Design review of the part built by this model. Coordinates are the model's own, in mm. A direction names the side the tool comes from. Give positions to 0.01 mm unless a question says otherwise; leave off trailing zeros. Write each loop counter-clockwise with the first axis right and the second up, starting at its lowest first coordinate (ties: lowest second). Pieces come first, ordered by that corner, then holes.
```python
from build123d import *

# Parameters (mm, degrees)
BOSS_EXTRUDE1_DEPTH = 14.478
BOSS_EXTRUDE2_DEPTH = 66.04
SKETCH3_W           = 80.518
SKETCH3_H           = 1.477027813
BOSS_EXTRUDE3_DEPTH = 1.524
SKETCH4_W           = 80.518
SKETCH4_H           = 1.559652671
CUT_EXTRUDE1_DEPTH  = 1.524
CUT_EXTRUDE3_DEPTH  = 14.478
CUT_EXTRUDE6_DEPTH  = 20.066


with BuildPart() as part:
    # Sketch1 → Boss-Extrude1 (new body)
    with BuildSketch(Plane.XY):
        with BuildLine():
            Line((-72.819716666, 29.55445925), (-5.08, 29.55445925))
            ThreePointArc((-5.08, 29.55445925), (-1.487897552, 28.066561699), (0, 24.47445925))
            Line((0, 24.47445925), (0, -4.589051483))
            ThreePointArc((0, -4.589051483), (-1.487897552, -8.181153932), (-5.08, -9.669051483))
            Line((-5.08, -9.669051483), (-72.819716666, -9.669051483))
            ThreePointArc((-72.819716666, -9.669051483), (-76.411819114, -8.181153932), (-77.899716666, -4.589051483))
            Line((-77.899716666, -4.589051483), (-77.899716666, 24.47445925))
            ThreePointArc((-77.899716666, 24.47445925), (-76.411819114, 28.066561699), (-72.819716666, 29.55445925))
        make_face()
        with BuildLine():
            Line((-65.339884386, 23.351671506), (-12.012527478, 23.351671506))
            ThreePointArc((-12.012527478, 23.351671506), (-8.42042503, 21.863773955), (-6.932527478, 18.271671506))
            Line((-6.932527478, 18.271671506), (-6.932527478, 3.07321573))
            ThreePointArc((-6.932527478, 3.07321573), (-8.42042503, -0.518886719), (-12.012527478, -2.00678427))
            Line((-12.012527478, -2.00678427), (-65.339884386, -2.00678427))
            ThreePointArc((-65.339884386, -2.00678427), (-68.931986835, -0.518886719), (-70.419884386, 3.07321573))
            Line((-70.419884386, 3.07321573), (-70.419884386, 18.271671506))
            ThreePointArc((-70.419884386, 18.271671506), (-68.931986835, 21.863773955), (-65.339884386, 23.351671506))
        make_face(mode=Mode.SUBTRACT)
    extrude(amount=BOSS_EXTRUDE1_DEPTH)

    # Sketch2 → Boss-Extrude2 (add)
    with BuildSketch(Plane(origin=(0, 0, 0), x_dir=(-1, 0, 0), z_dir=(0, 0, -1))):
        with BuildLine():
            Line((5.08, 29.55445925), (72.819716666, 29.55445925))
            ThreePointArc((72.819716666, 29.55445925), (76.411819114, 28.066561699), (77.899716666, 24.47445925))
            Line((77.899716666, 24.47445925), (77.899716666, -4.589051483))
            ThreePointArc((77.899716666, -4.589051483), (76.411819114, -8.181153932), (72.819716666, -9.669051483))
            Line((72.819716666, -9.669051483), (5.08, -9.669051483))
            ThreePointArc((5.08, -9.669051483), (1.487897552, -8.181153932), (0, -4.589051483))
            Line((0, -4.589051483), (0, 24.47445925))
            ThreePointArc((0, 24.47445925), (1.487897552, 28.066561699), (5.08, 29.55445925))
        make_face()
    extrude(amount=BOSS_EXTRUDE2_DEPTH)

    # Sketch3 → Boss-Extrude3 (add)
    with BuildSketch(Plane.ZY.offset(77.899716666)):
        with Locations((-25.781, 23.735945344)):
            Rectangle(SKETCH3_W, SKETCH3_H)
    extrude(amount=-BOSS_EXTRUDE3_DEPTH)

    # Sketch4 → Cut-Extrude1 (cut)
    with BuildSketch(Plane.ZY.offset(77.899716666)):
        with Locations((-25.781, 23.694632915)):
            Rectangle(SKETCH4_W, SKETCH4_H)
    extrude(amount=-CUT_EXTRUDE1_DEPTH, mode=Mode.SUBTRACT)

    # Sketch8 → Cut-Extrude3 (cut)
    with BuildSketch(Plane(origin=(0, 0.399775278, -66.04), x_dir=(-1, 0, 0), z_dir=(0, 0, -1))):
        with BuildLine():
            Line((13.813270209, 22.173227648), (64.646012904, 22.173227648))
            ThreePointArc((64.646012904, 22.173227648), (68.238115352, 20.685330097), (69.726012904, 17.093227648))
            Line((69.726012904, 17.093227648), (69.726012904, 3.751436885))
            ThreePointArc((69.726012904, 3.751436885), (68.238115352, 0.159334436), (64.646012904, -1.328563115))
            Line((64.646012904, -1.328563115), (13.813270209, -1.328563115))
            ThreePointArc((13.813270209, -1.328563115), (10.22116776, 0.159334436), (8.733270209, 3.751436885))
            Line((8.733270209, 3.751436885), (8.733270209, 17.093227648))
            ThreePointArc((8.733270209, 17.093227648), (10.22116776, 20.685330097), (13.813270209, 22.173227648))
        make_face()
    extrude(amount=-CUT_EXTRUDE3_DEPTH, mode=Mode.SUBTRACT)

    # Sketch10 → Cut-Extrude6 (cut)
    with BuildSketch(Plane(origin=(0, 29.55445925, 6.792687041), x_dir=(1, 0, 0), z_dir=(0, 1, 0))):
        with BuildLine():
            Line((-65.795513853, 57.457874707), (-12.761974665, 57.457874707))
            ThreePointArc((-12.761974665, 57.457874707), (-9.169872217, 55.969977155), (-7.681974665, 52.377874707))
            Line((-7.681974665, 52.377874707), (-7.681974665, 11.913822303))
            ThreePointArc((-7.681974665, 11.913822303), (-9.169872217, 8.321719854), (-12.761974665, 6.833822303))
            Line((-12.761974665, 6.833822303), (-65.795513853, 6.833822303))
            ThreePointArc((-65.795513853, 6.833822303), (-69.387616301, 8.321719854), (-70.875513853, 11.913822303))
            Line((-70.875513853, 11.913822303), (-70.875513853, 52.377874707))
            ThreePointArc((-70.875513853, 52.377874707), (-69.387616301, 55.969977155), (-65.795513853, 57.457874707))
        make_face()
    extrude(amount=-CUT_EXTRUDE6_DEPTH, mode=Mode.SUBTRACT)


solid = part.part
```
(1) To check wall thickness, follow L1, parallel to Z at x = -61, y = 26; L2, parallel to X at y = 11, z = -18.5; L3, parallel to Y at x = -38.5, z = 5. State the ranges of each line that lie inside material, in increasing order.
Resolved:
L1: z = -66.04 to -50.67, -0.04 to 14.48
L2: x = -77.9 to -70.88, -7.68 to 0
L3: y = -9.67 to -2.01, 23.35 to 29.55
(2) Tool access review of faces 1 (the face through (-68.198, 21.124, -58.902)), 2 (the face through (-8.4, -0.5, 7.1)), 3 (the face through (-69.35, 19.66, -1.49)): name each direction out of +Z, -Z, +X, -X, +Y, -Y from which nothing blocks a thin tool from reaching the whole face with its end or side.
Resolved:
face 1: -Z
face 2: +Z
face 3: +Y
(3) Consider section C-C, the plane x = -55. Give the boundary of the cut face in (y, z).
Resolved:
outline: (-9.67, -66.04) - (-0.93, -66.04) - (-0.93, -51.56) - (22.57, -51.56) - (22.57, -66.04) - (29.55, -66.04) - (29.55, -50.67) - (9.49, -50.67) - (9.49, -0.04) - (29.55, -0.04) - (29.55, 14.48) - (23.35, 14.48) - (23.35, 0) - (-2.01, 0) - (-2.01, 14.48) - (-9.67, 14.48) - close
(4) Consider section A-A, the plane z = -19. Give the boundary of the cut face in (x, y).
Resolved:
outline: (-77.9, -4.59) arc R5.08 ccw to (-72.82, -9.67) - (-5.08, -9.67) arc R5.08 ccw to (0, -4.59) - (0, 24.47) arc R5.08 ccw to (-5.08, 29.55) - (-7.68, 29.55) - (-7.68, 9.49) - (-70.88, 9.49) - (-70.88, 29.55) - (-72.82, 29.55) arc R5.08 ccw to (-77.9, 24.47) - (-76.38, 24.47) - (-76.38, 22.91) - (-77.9, 22.91) - close
(5) Consider section D-D, the plane y = 0.5. Give the boundary of the cut face in (x, z), then the cut area to 3 significant figures.
Resolved:
outline: (-77.9, -66.04) - (-68.18, -66.04) - (-68.18, -51.56) - (-10.28, -51.56) - (-10.28, -66.04) - (0, -66.04) - (0, 14.48) - (-7.63, 14.48) - (-7.63, 0) - (-69.72, 0) - (-69.72, 14.48) - (-77.9, 14.48) - close
area: 4,540 mm2
(6) Clearance check with flat-ended pins moving along their axes: P1, Ø4, axis at x = -64, y = 9.5, coming from the -Z side; P2, Ø4, axis at x = -45, z = -35, coming from the +Y side; P3, Ø1.2, axis at x = -77, z = -20, coming from the -Y side. State where each tip first meets the part, or that it passes through.
Resolved:
P1: stops at z = -51.56
P2: stops at y = 9.49
P3: stops at y = -8.19
(7) Mouldability with a two-part tool opening along Y and no side actions: class faces 4 (the face through (0, 10, -25)), 5 (the face through (-40, 11, -51.562)), 6 (the face through (-76.45, -8.14, -25.22)), 7 (the face through (-1.45, 28.03, -25.22)) as pulls with the +Y half, pulls with the -Y half, needs draft (parallel to the pull), parting line crosses it, or undercut.
Resolved:
face 4: needs draft
face 5: undercut
face 6: pulls with the -Y half
face 7: pulls with the +Y half
(8) Consider section B-B, the plane z = 3. Give the boundary of the cut face in (x, y), then the cut area to 3 significant figures.
Resolved:
outline: (-77.9, -4.59) arc R5.08 ccw to (-72.82, -9.67) - (-5.08, -9.67) arc R5.08 ccw to (0, -4.59) - (0, 24.47) arc R5.08 ccw to (-5.08, 29.55) - (-72.82, 29.55) arc R5.08 ccw to (-77.9, 24.47) - (-76.38, 24.47) - (-76.38, 22.91) - (-77.9, 22.91) - close; hole (-70.42, 3.07) arc R5.08 ccw to (-65.34, -2.01) - (-12.01, -2.01) arc R5.08 ccw to (-6.93, 3.07) - (-6.93, 18.27) arc R5.08 ccw to (-12.01, 23.35) - (-65.34, 23.35) arc R5.08 ccw to (-70.42, 18.27) - close
area: 1,440 mm2
